```python
from build123d import *

# Parameters (mm, degrees)
F0_W          = 50
F0_H          = 50
F0_W_2        = 45
F0_H_2        = 45
F1_DEPTH      = 200
F2_W          = 50
F2_H          = 50
F2_W_2        = 45
F2_H_2        = 45
F3_DEPTH      = 700
F4_W          = 20
F4_H          = 20
F4_W_2        = 17
F4_H_2        = 17
F5_DEPTH      = 50
F6_DEPTH      = 50
F7_W          = 20
F7_H          = 20
F7_W_2        = 17
F7_H_2        = 17
F8_DEPTH      = 535
F9_R          = 6
F10_DEPTH     = 750.001
F11_R         = 13
F11_R_2       = 11
F12_DEPTH     = 10
F13_DEPTH     = 5
F14_R         = 13
F14_R_2       = 11
F15_DEPTH     = 10
F16_DEPTH     = 5
F17_T4_ANGLE  = 213.9701071651
F17_T10_ANGLE = 213.9701071651
F17_T16_ANGLE = 213.9701071651
F17_T22_ANGLE = 213.9701071651
F18_R         = 2.5
F19_DEPTH     = 10


# Not quite as in the source:
# - a fillet or chamfer that OpenCascade refuses, or shapes differently, is made with other operations: its cross-section is extruded or revolved along the edge and cut away or added


with BuildPart() as f1:
    # F0 (on Front) → F1 (new body, symmetric)
    with BuildSketch(Plane.XZ):
        with Locations((-375, 0)):
            Rectangle(F0_W, F0_H)
        with Locations((-375, 0)):
            Rectangle(F0_W_2, F0_H_2, mode=Mode.SUBTRACT)
    extrude(amount=F1_DEPTH, both=True)



with BuildPart() as f1b:
    # F0 (on Front) → F1, piece 2 (new body, symmetric)
    with BuildSketch(Plane.XZ):
        with Locations((375, 0)):
            Rectangle(F0_W, F0_H)
        with Locations((375, 0)):
            Rectangle(F0_W_2, F0_H_2, mode=Mode.SUBTRACT)
    extrude(amount=F1_DEPTH, both=True)


with BuildPart() as f1_1:
    add(f1.part)

    add(f1b.part)  # F3 merges F1b
    # F2 (on face) → F3 (join, through all)
    with BuildSketch(Plane.YZ.offset(-350)):
        with Locations((50, 0)):
            Rectangle(F2_W, F2_H)
        with Locations((50, 0)):
            Rectangle(F2_W_2, F2_H_2, mode=Mode.SUBTRACT)
        with Locations((-50, 0)):
            Rectangle(F2_W, F2_H)
        with Locations((-50, 0)):
            Rectangle(F2_W_2, F2_H_2, mode=Mode.SUBTRACT)
    extrude(amount=F3_DEPTH)

    # F4 (on face) → F5 (join)
    with BuildSketch(Plane.XY.offset(25)):
        with Locations((340, -85)):
            Rectangle(F4_W, F4_H)
        with Locations((340, -85)):
            Rectangle(F4_W_2, F4_H_2, mode=Mode.SUBTRACT)
        with Locations((-175, -85)):
            Rectangle(F4_W, F4_H)
        with Locations((-175, -85)):
            Rectangle(F4_W_2, F4_H_2, mode=Mode.SUBTRACT)
    extrude(amount=-F5_DEPTH)

    # F4 (on face) → F6 (join)
    with BuildSketch(Plane.XY.offset(25)):
        with Locations((340, -85)):
            Rectangle(F4_W, F4_H)
        with Locations((340, -85)):
            Rectangle(F4_W_2, F4_H_2, mode=Mode.SUBTRACT)
        with Locations((-175, -85)):
            Rectangle(F4_W, F4_H)
        with Locations((-175, -85)):
            Rectangle(F4_W_2, F4_H_2, mode=Mode.SUBTRACT)
    extrude(amount=F6_DEPTH)

    # F7 (on face) → F8 (join)
    with BuildSketch(Plane(origin=(350, 0, 0), x_dir=(0, -1, 0), z_dir=(-1, 0, 0))):
        with Locations((105, 15)):
            Rectangle(F7_W, F7_H)
        with Locations((105, 15)):
            Rectangle(F7_W_2, F7_H_2, mode=Mode.SUBTRACT)
    extrude(amount=F8_DEPTH)

    # F9 (on face) → F10 (cut, through all)
    with BuildSketch(Plane.YZ.offset(350)):
        with Locations((-85, 50)):
            Circle(F9_R)
    extrude(amount=-F10_DEPTH, mode=Mode.SUBTRACT)

    # F11 (on face) → F12 (join)
    with BuildSketch(Plane(origin=(330, 0, 0), x_dir=(0, -1, 0), z_dir=(-1, 0, 0))):
        with Locations((85, 50)):
            Circle(F11_R)
        with Locations((85, 50)):
            Circle(F11_R_2, mode=Mode.SUBTRACT)
    extrude(amount=F12_DEPTH)

    # F11 (on face) → F13 (join)
    with BuildSketch(Plane(origin=(330, 0, 0), x_dir=(0, -1, 0), z_dir=(-1, 0, 0))):
        with Locations((85, 50)):
            Circle(F11_R)
        with Locations((85, 50)):
            Circle(F11_R_2, mode=Mode.SUBTRACT)
    extrude(amount=-F13_DEPTH)

    # F14 (on face) → F15 (join)
    with BuildSketch(Plane.YZ.offset(-165)):
        with Locations((-85, 50)):
            Circle(F14_R)
        with Locations((-85, 50)):
            Circle(F14_R_2, mode=Mode.SUBTRACT)
    extrude(amount=F15_DEPTH)

    # F14 (on face) → F16 (join)
    with BuildSketch(Plane.YZ.offset(-165)):
        with Locations((-85, 50)):
            Circle(F14_R)
        with Locations((-85, 50)):
            Circle(F14_R_2, mode=Mode.SUBTRACT)
    extrude(amount=-F16_DEPTH)

    # F17: chamfer of 5 on 10 edges, made by hand


with BuildPart() as f17_tool2:
    # F17_s3 → F17_t4 (revolve)
    with BuildSketch(Plane(origin=(0, 6.7154986509, 21.9859176279), x_dir=(1, 0, 0), z_dir=(0, 0.2921222291, 0.9563809927))):
        Polygon((-165, -113.8984958377), (-160, -108.8984958377), (-165, -108.8984958377), align=None)
    revolve(axis=Axis((-165, -85, 50), (1, 0, 0)), revolution_arc=F17_T4_ANGLE)

    split(bisect_by=Plane.XZ.offset(75), keep=Keep.TOP)

    split(bisect_by=Plane.XZ.offset(95), keep=Keep.BOTTOM)


with BuildPart() as f1_2:
    add(f1_1.part)

    # F17_t1: union F17_tool2
    add(f17_tool2.part)


with BuildPart() as f17_tool8:
    # F17_s9 → F17_t10 (revolve)
    with BuildSketch(Plane(origin=(0, 6.7154986509, 21.9859176279), x_dir=(1, 0, 0), z_dir=(0, -0.2921222291, -0.9563809927))):
        Polygon((-165, 77.8984958377), (-160, 82.8984958377), (-165, 82.8984958377), align=None)
    revolve(axis=Axis((-165, -85, 50), (1, 0, 0)), revolution_arc=F17_T10_ANGLE)

    split(bisect_by=Plane.XZ.offset(75), keep=Keep.TOP)

    split(bisect_by=Plane.XZ.offset(95), keep=Keep.BOTTOM)


with BuildPart() as f1_3:
    add(f1_2.part)

    # F17_t7: union F17_tool8
    add(f17_tool8.part)


with BuildPart() as f17_tool14:
    # F17_s15 → F17_t16 (revolve)
    with BuildSketch(Plane(origin=(0, -21.2225160964, 69.4805426982), x_dir=(1, 0, 0), z_dir=(0, -0.2921222291, 0.9563809927))):
        Polygon((330, -48.686272927), (325, -53.686272927), (330, -53.686272927), align=None)
    revolve(axis=Axis((330, -85, 50), (-1, 0, 0)), revolution_arc=F17_T16_ANGLE)

    split(bisect_by=Plane.XZ.offset(75), keep=Keep.TOP)

    split(bisect_by=Plane.XZ.offset(95), keep=Keep.BOTTOM)


with BuildPart() as f1_4:
    add(f1_3.part)

    # F17_t13: union F17_tool14
    add(f17_tool14.part)


with BuildPart() as f17_tool20:
    # F17_s21 → F17_t22 (revolve)
    with BuildSketch(Plane(origin=(0, -21.2225160964, 69.4805426982), x_dir=(1, 0, 0), z_dir=(0, 0.2921222291, -0.9563809927))):
        Polygon((330, 84.686272927), (325, 79.686272927), (330, 79.686272927), align=None)
    revolve(axis=Axis((330, -85, 50), (-1, 0, 0)), revolution_arc=F17_T22_ANGLE)

    split(bisect_by=Plane.XZ.offset(75), keep=Keep.TOP)

    split(bisect_by=Plane.XZ.offset(95), keep=Keep.BOTTOM)


with BuildPart() as f1_5:
    add(f1_4.part)

    # F17_t19: union F17_tool20
    add(f17_tool20.part)

    # F18 (on face) → F19 (cut)
    with BuildSketch(Plane.XY.offset(25)):
        with Locations((-175, -65)):
            Circle(F18_R)
        with Locations((-175, 65)):
            Circle(F18_R)
        with Locations((-175, -105)):
            Circle(F18_R)
        with Locations((340, -105)):
            Circle(F18_R)
        with Locations((340, -65)):
            Circle(F18_R)
        with Locations((340, 65)):
            Circle(F18_R)
    extrude(amount=-F19_DEPTH, mode=Mode.SUBTRACT)


solid = f1_5.part
```
Here's how the part is built. I have some questions about the finished solid (model axes, mm). A direction names the side the tool comes from. Give positions to 0.01 mm unless a question says otherwise; leave off trailing zeros. Order: outer loops, then holes, each group sorted by start corner. A loop starts at its lowest first (then second) coordinate and runs counter-clockwise, first axis right, second up. Notation, with made-up numbers: (26, 85.5) -> (78, 85.5) arc R13 cw to (78, 103.5) -> close; hole circle Ø8 at (-36, 17). An arc over 180 degrees is marked (long way). Use CSV: the item, a comma, the result in double quotes. Start each with the question number.
Item 1: Suppose I cut it at C-C (y = 126). List the corners of the cut face in (x, z) for me, and give its area (3 significant figures).
Item 2: If I drill on probe 1 along X at (y, z) = (-4.5, 0.5); probe 2 along Y at (x, z) = (105, -7); probe 3 along Y at (x, z) = (340, 24.1), over which ranges is the centre line in solid material (lowest first)? Write a range as [from, to].
Item 3: Suppose I cut it at B-B (x = -80). List the corners of the cut face in (y, z) for me.
Item 4: Suppose I cut it at A-A (x = -212). List the corners of the cut face in (y, z) for me.
Item 5: Thinking about a two-plate mould opening in X: for faces 4 (the flat face through (-166, -85, 75)), 5 (the flat face through (-400, -3, 0)), 6 (the flat face through (-350, -50, 0)), which applies, pulls with the +X half, pulls with the -X half, needs draft (parallel to the pull), parting line crosses it, or undercut?
Item 6: On a 3-axis mill with a long thin cutter (end or side, diameter ignored), from which of +Z, -Z, +X, -X, +Y, -Y can I reach the whole of each face in a straight line? I mean faces 1 (the flat face through (350, -105, 15)), 2 (the flat face through (-175, -95, -10)), 3 (the flat face through (-5, 75, 0)). Say none if no direction works.
Item 7: I'm going to push flat-ended pins straight in: P1, Ø20, axis at x = -177, z = 60.5, coming from the -Y side; P2, Ø22, axis at x = -178, z = -7, coming from the -Y side; P3, Ø6, axis at x = -43, y = -71, coming from the +Z side. Where does each tip first touch, or does it pass through?
Answer block:
1,outline,"(-400, -25) -> (-350, -25) -> (-350, 25) -> (-400, 25) -> close; (350, -25) -> (400, -25) -> (400, 25) -> (350, 25) -> close; hole (-397.5, -22.5) -> (-352.5, -22.5) -> (-352.5, 22.5) -> (-397.5, 22.5) -> close; hole (352.5, -22.5) -> (397.5, -22.5) -> (397.5, 22.5) -> (352.5, 22.5) -> close"
1,area,"950 mm^2"
2,probe 1,"x = [-400, -397.5], [-352.5, -350], [350, 352.5], [397.5, 400]"
2,probe 2,"y = [-75, -72.5], [-27.5, -25], [25, 27.5], [72.5, 75]"
2,probe 3,"y = [-115, -107.5], [-102.5, -93.5], [-76.5, -67.5], [-62.5, -25], [25, 62.5], [67.5, 75]"
3,outline,"(-115, 5) -> (-95, 5) -> (-95, 25) -> (-115, 25) -> close; (-75, -25) -> (-25, -25) -> (-25, 25) -> (-75, 25) -> close; (25, -25) -> (75, -25) -> (75, 25) -> (25, 25) -> close; hole (-113.5, 6.5) -> (-96.5, 6.5) -> (-96.5, 23.5) -> (-113.5, 23.5) -> close; hole (-72.5, -22.5) -> (-27.5, -22.5) -> (-27.5, 22.5) -> (-72.5, 22.5) -> close; hole (27.5, -22.5) -> (72.5, -22.5) -> (72.5, 22.5) -> (27.5, 22.5) -> close"
4,outline,"(-75, -25) -> (-25, -25) -> (-25, 25) -> (-75, 25) -> close; (25, -25) -> (75, -25) -> (75, 25) -> (25, 25) -> close; hole (-72.5, -22.5) -> (-27.5, -22.5) -> (-27.5, 22.5) -> (-72.5, 22.5) -> close; hole (27.5, -22.5) -> (72.5, -22.5) -> (72.5, 22.5) -> (27.5, 22.5) -> close"
5,face 4,"needs draft"
5,face 5,"pulls with the -X half"
5,face 6,"undercut"
6,face 1,"none"
6,face 2,"-Z, -Y"
6,face 3,"+Z, -Z, +Y"
7,P1,"stops at y = -97.56"
7,P2,"stops at y = -95"
7,P3,"stops at z = 25"
